Autodesk Inventor part; units mm, degrees
ref_plane "YZ Plane" through (0, 0, 0) normal (1, 0, 0) x (0, 1, 0)
ref_plane "XZ Plane" through (0, 0, 0) normal (0, 1, 0) x (-1, 0, 0)
ref_plane "XY Plane" through (0, 0, 0) normal (0, 0, 1) x (1, 0, 0)
sketch "スケッチ1" plane through (0, 0, 0) normal (0, 0, 1) x (1, 0, 0)
  line L0 (-25, 12.5) -> (25, 12.5)
  line L1 (25, 12.5) -> (25, -12.5)
  line L2 (25, -12.5) -> (-25, -12.5)
  line L3 (-25, -12.5) -> (-25, 12.5)
  line L4 (-23, 10.5) -> (23, 10.5)
  line L5 (23, 10.5) -> (23, -10.5)
  line L6 (23, -10.5) -> (-23, -10.5)
  line L7 (-23, -10.5) -> (-23, 10.5)
  point P0 (0, 0)
  dimension "d0" = 50
  dimension "d2" = 25
  dimension "d3" = 21
  dimension "d4" = 46
  dimension "d5" = 23
  dimension "d6" = 25
  dimension "d7" = 10.5
  dimension "d8" = 12.5
extrude "押し出し1" add sketch "スケッチ1" against normal blind 225
sketch "スケッチ2" plane through (25, -12.5, 0) normal (1, 0, 0) x (0, 0, -1)
  line L0 (0, 0) -> (225, 0)
  line L1 (225, 25) -> (225, 0)
  circle A0 centre (181, 15) radius 2
  circle A1 centre (211, 9) radius 2
  point P0 (0, 12.5)
  dimension "d11" = 4
  dimension "d13" = 30
  dimension "d16" = 14
  dimension "d17" = 9
  dimension "d61" = 15
hole "穴1" at (25, -3.5, -211) at (25, 2.5, -181) direction (-1, 0, 0) diameter 4 end through all
sketch "スケッチ3" plane through (25, -12.5, 0) normal (1, 0, 0) x (0, 0, -1)
  line L0 (0, 25) -> (0, 0)
  line L1 (0, 0) -> (225, 0)
  circle A0 centre (10.5, 12.5) radius 2
  point P0 (0, 12.5)
  dimension "d25" = 4
  dimension "d27" = 12.5
  dimension "d28" = 10.5
hole "穴2" at (25, 0, -10.5) direction (-1, 0, 0) diameter 4 end through all
sketch "スケッチ4" plane through (25, -12.5, 0) normal (1, 0, 0) x (0, 0, -1)
  circle A0 centre (10.5, 12.5) radius 2
  line L0 (0, 25) -> (0, 0)
  line L1 (0, 19) -> (33.5, 19)
  line L2 (33.5, 6) -> (0, 6)
  line L3 (0, 6) -> (0, 19)
  arc A1 (33.5, 6) -> (33.5, 19) centre (33.5, 12.5) ccw
  point P0 (0, 12.5)
  dimension "d36" = 13
  dimension "d38" = 6.5
  dimension "d39" = 13
  dimension "d40" = 33.5
extrude "押し出し2" cut sketch "スケッチ4" against normal blind 2
sketch "スケッチ5" plane through (25, -12.5, -225) normal (1, 0, 0) x (0, 0, -1)
  arc A0 (-191.5, 6) -> (-191.5, 19) centre (-191.5, 12.5) ccw
  line L0 (-225, 6) -> (-225, 0)
  line L1 (-225, 25) -> (-225, 19)
  circle A1 centre (-221, 4.5) radius 1
  circle A2 centre (-221, 20.5) radius 1
  circle A3 centre (-185, 20.5) radius 1
  circle A4 centre (-185, 4.5) radius 1
  point P0 (-225, 12.5)
  dimension "d43" = 36
  dimension "d45" = 36
  dimension "d46" = 16
  dimension "d47" = 8
  dimension "d48" = 2
  dimension "d49" = 16
  dimension "d50" = 8
  dimension "d51" = 4
  dimension "d52" = 4
hole "穴3" at (25, 8, -4) at (25, -8, -4) at (25, -8, -40) at (25, 8, -40) direction (-1, 0, 0) diameter 2 depth 2 tip angle 118 counterbore diameter 4 counterbore depth 0.5
properties part number "Arm_Second_Flame"
Verification items for the finished model (mm, model axes). A direction names the side the tool comes from. Give positions to 0.01 mm unless a question says otherwise; leave off trailing zeros. Order: outer loops, then holes, each group sorted by start corner. A loop starts at its lowest first (then second) coordinate and runs counter-clockwise, first axis right, second up. Notation, with made-up numbers: (79, -4) -> (104, -4) arc R5 ccw to (104, 0) -> close; hole circle Ø10 at (28.25, 64). An arc over 180 degrees is marked (long way). One line per item, written item: value.
(1) Gauge pin test, flat ends, axial feed: pin 1 (3 mm diameter, centred on y = -8, z = -4, fed in from +X); pin 2 (6.5 mm diameter, centred on y = 0, z = -10.5, fed in from +X). Record the tip position at first contact, or that the pin passes through.
Final values:
pin 1: x = 24.5
pin 2: x = -23
(2) Sectioned sample at B-B on z = -173.5. Record the cut outline in (x, y), then the cut area to 3 significant figures.
Final values:
outline: (-25, -12.5) -> (25, -12.5) -> (25, 12.5) -> (-25, 12.5) -> close; hole (-23, -10.5) -> (23, -10.5) -> (23, 10.5) -> (-23, 10.5) -> close
area: 284 mm^2
(3) Draft check along Z on faces 4 (the face through (24, 0, -40)), 5 (the face through (0, 12.5, -111)), 6 (the face through (24.5, -7, -41)). Enter one of: pulls with the +Z half, pulls with the -Z half, needs draft (parallel to the pull), parting line crosses it, or undercut.
Final values:
face 4: pulls with the +Z half
face 5: needs draft
face 6: undercut
(4) Sectioned sample at C-C on z = -10.5. Record the cut outline in (x, y), then the cut area to 3 significant figures.
Final values:
outline: (-25, -12.5) -> (25, -12.5) -> (25, -6.5) -> (23, -6.5) -> (23, -10.5) -> (-23, -10.5) -> (-23, -2) -> (-25, -2) -> close; (-25, 2) -> (-23, 2) -> (-23, 10.5) -> (23, 10.5) -> (23, 6.5) -> (25, 6.5) -> (25, 12.5) -> (-25, 12.5) -> close
area: 250 mm^2
(5) Tool access check on faces 1 (the face through (24.5, 9, -5)), 2 (the face through (-23, 0, -111)), 3 (the face through (23.986, 2.412, -179.002)). Record the directions out of +Z, -Z, +X, -X, +Y, -Y that give a thin tool (end or side, any length) a straight path to the whole face; none if there is none.
Final values:
face 1: +X
face 2: +Z, -Z
face 3: +X, -X
(6) Sectioned sample at A-A on x = -14.5. Record the cut outline in (y, z), then the cut area to 3 significant figures.
Final values:
outline: (-12.5, -225) -> (-10.5, -225) -> (-10.5, 0) -> (-12.5, 0) -> close; (10.5, -225) -> (12.5, -225) -> (12.5, 0) -> (10.5, 0) -> close
area: 900 mm^2
(7) Scan lines: line 1 along Y through (x, z) = (-4, -117); line 2 along X through (y, z) = (6, -154); line 3 along Y through (x, z) = (24.5, -211). Record each from-to range of solid material in increasing order. Write a range as [from, to].
Final values:
line 1: [-12.5, -10.5], [10.5, 12.5]
line 2: [-25, -23], [23, 25]
line 3: [-12.5, -5.5], [-1.5, 12.5]
